CAD build for the part. Positions are in the model's coordinates, mm. A direction names the side the tool comes from. Round coordinates to 2 decimals unless told otherwise and drop trailing zeros. Loops run counter-clockwise (first coordinate to the right, second up) from the corner with the lowest first, then second, coordinate; pieces in that order, holes last. Notation, with made-up numbers: M 64,61.25 L 101,61.25 A25 ccw 101,83.25 Z; hole C 66,-14.75 d2. An arc over 180 degrees is marked long. One line per item, written item: value. Start each with the question number.
from build123d import *

# Parameters (mm, degrees)
F1_DEPTH = 25.4
F2_W     = 107.5181365013
F2_H     = 53.2084149309
F3_DEPTH = 50.8
F4_R     = 43.6587817112
F5_DEPTH = 203.2


with BuildPart() as f1:
    # F0 (on Front) → F1 (new body)
    with BuildSketch(Plane.XZ):
        with BuildLine():
            Line((-103.3638969086, 22.86), (-103.3638969086, 38.1))
            ThreePointArc((-103.3638969086, 38.1), (-141.4638969086, 0), (-103.3638969086, -38.1))
            Line((-103.3638969086, -38.1), (-103.3638969086, -22.86))
            ThreePointArc((-103.3638969086, -22.86), (-126.2238969086, 0), (-103.3638969086, 22.86))
        make_face()
        with BuildLine():
            ThreePointArc((141.4638969086, 0), (130.3046652718, 26.9407683632), (103.3638969086, 38.1))
            Line((103.3638969086, 38.1), (103.3638969086, 22.86))
            ThreePointArc((103.3638969086, 22.86), (119.5283579265, 16.1644610179), (126.2238969086, 0))
            ThreePointArc((126.2238969086, 0), (119.5283579265, -16.1644610179), (103.3638969086, -22.86))
            Line((103.3638969086, -22.86), (103.3638969086, -38.1))
            ThreePointArc((103.3638969086, -38.1), (130.3046652718, -26.9407683632), (141.4638969086, 0))
        make_face()
        with BuildLine():
            ThreePointArc((-65.2638969086, 0), (-76.4231285454, 26.9407683632), (-103.3638969086, 38.1))
            Line((-103.3638969086, 38.1), (-103.3638969086, 22.86))
            ThreePointArc((-103.3638969086, 22.86), (-87.1994358907, 16.1644610179), (-80.5038969086, 0))
            ThreePointArc((-80.5038969086, 0), (-87.1994358907, -16.1644610179), (-103.3638969086, -22.86))
            Line((-103.3638969086, -22.86), (-103.3638969086, -38.1))
            ThreePointArc((-103.3638969086, -38.1), (-76.4231285454, -26.9407683632), (-65.2638969086, 0))
        make_face()
        with BuildLine():
            Line((103.3638969086, 22.86), (103.3638969086, 38.1))
            ThreePointArc((103.3638969086, 38.1), (65.2638969086, 0), (103.3638969086, -38.1))
            Line((103.3638969086, -38.1), (103.3638969086, -22.86))
            ThreePointArc((103.3638969086, -22.86), (80.5038969086, 0), (103.3638969086, 22.86))
        make_face()
        with BuildLine():
            Line((103.3638969086, 38.1), (-103.3638969086, 38.1))
            ThreePointArc((-103.3638969086, 38.1), (-76.4231285454, 26.9407683632), (-65.2638969086, 0))
            ThreePointArc((-65.2638969086, 0), (-76.4231285454, -26.9407683632), (-103.3638969086, -38.1))
            Line((-103.3638969086, -38.1), (103.3638969086, -38.1))
            ThreePointArc((103.3638969086, -38.1), (65.2638969086, 0), (103.3638969086, 38.1))
        make_face()
    extrude(amount=F1_DEPTH)

    # F2 (on face) → F3 (join)
    with BuildSketch(Plane.XZ.offset(25.4)):
        with Locations((0, -1.8939918373)):
            Rectangle(F2_W, F2_H)
    extrude(amount=F3_DEPTH)

    # F4 (on face) → F5 (cut)
    with BuildSketch(Plane(origin=(0, 0, -28.4981993027), x_dir=(1, 0, 0), z_dir=(0, 0, -1))):
        with Locations((0, 76.2)):
            Circle(F4_R)
    extrude(amount=-F5_DEPTH, mode=Mode.SUBTRACT)


solid = f1.part
(1) Flat gauge pins, fed straight in: P1, Ø2, axis at y = -35.5, z = 13, coming from the -X side; P2, Ø4, axis at y = -16, z = 17.5, coming from the +X side; P3, Ø3, axis at y = -24.5, z = -27, coming from the +X side. Where does each tip first touch, or does it go through?
(2) Which spindle directions (+Z, -Z, +X, -X, +Y, -Y) get a long thin tool onto all of the face, cutting with end or side? Do faces 4 (the flat face through (53.759, -50, -2)), 5 (the flat face through (-13, -34, -28.498)), 6 (the flat face through (-13, -34, 24.71)). Say none if no direction does.
(3) Slice it at A-A, the plane y = -15.5. List the corners of the cut face in (x, z).
(4) Slice it at B-B, the plane z = -19.5. List the corners of the cut face in (x, y), and give its area (3 significant figures).
(5) Mould opens along X. For faces 1 (the cylindrical face through (-0.96, -32.55, -2.27)), 2 (the flat face through (-53.759, -50, -2)), 3 (the flat face through (-49, -76.2, -2)) say: pulls with the +X half, pulls with the -X half, needs draft (parallel to the pull), parting line crosses it, or undercut.
(6) Slice it at C-C, the plane y = -51.5. List the corners of the cut face in (x, z).
(7) Probe L1, parallel to X at y = -12.5, z = 15; L2, parallel to X at y = -11.5, z = 13; L3, parallel to Y at x = 73.5, z = -20. List the from-to ranges inside material, lowest first.
(8) Slice it at D-D, the plane x = 92. List the corners of the cut face in (y, z).
Check result:
1. P1: stops at x = -53.76
1. P2: stops at x = 138.17
1. P3: stops at x = 131.67
2. face 4: +Z, -Z, +X, -Y
2. face 5: -Z, +X, -X, -Y
2. face 6: +Z, +X, -X, -Y
3. outline: M -103.36,-38.1 L 103.36,-38.1 A38.1 ccw 103.36,38.1 L -103.36,38.1 A38.1 ccw Z; hole C -103.36,0 d45.72; hole C 103.36,0 d45.72
4. outline: M -136.1,-25.4 L -115.29,-25.4 L -115.29,0 L -136.1,0 Z; M -91.43,-25.4 L -53.76,-25.4 L -53.76,-76.2 L -43.66,-76.2 A43.66 cw 43.66,-76.2 L 53.76,-76.2 L 53.76,-25.4 L 91.43,-25.4 L 91.43,0 L -91.43,0 Z; M 115.29,-25.4 L 136.1,-25.4 L 136.1,0 L 115.29,0 Z
4. area: 8,170 mm^2
5. face 1: undercut
5. face 2: pulls with the -X half
5. face 3: needs draft
6. outline: M -53.76,-28.5 L -36,-28.5 L -36,24.71 L -53.76,24.71 Z; M 36,-28.5 L 53.76,-28.5 L 53.76,24.71 L 36,24.71 Z
7. L1: x = -138.39 to -120.61, -86.11 to 86.11, 120.61 to 138.39
7. L2: x = -139.18 to -122.17, -84.56 to 84.56, 122.17 to 139.18
7. L3: y = -25.4 to 0
8. outline: M -25.4,-38.1 L 0,-38.1 L 0,-19.84 L -25.4,-19.84 Z; M -25.4,19.84 L 0,19.84 L 0,38.1 L -25.4,38.1 Z
